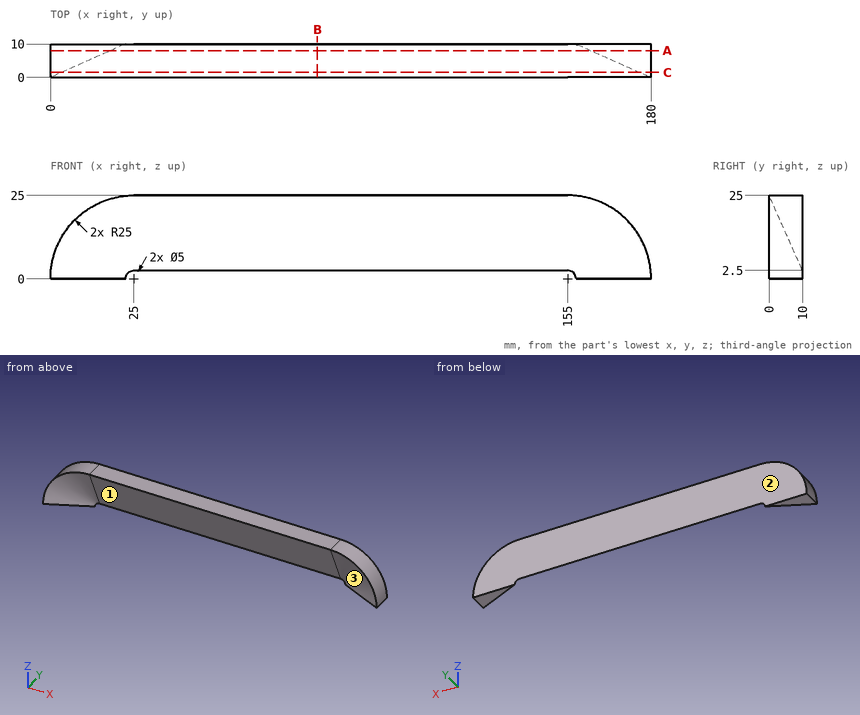
The drawing under review shows one solid part. Ordinate dimensions are in mm from its lowest x, y, z. Give positions to 0.01 mm unless a question says otherwise; leave off trailing zeros. Order: outer loops, then holes, each group sorted by start corner. A loop starts at its lowest first (then second) coordinate and runs counter-clockwise, first axis right, second up. Notation, with made-up numbers: (-33.5, 10) - (0.5, 10) arc R22 cw to (0.5, 27) - close; hole circle Ø1 at (75.25, 25.5). An arc over 180 degrees is marked (long way). Answer as a JSON object with one key per item and string values. Group by question number.
Item 1: Wall thickness on line 1 along X through (y, z) = (1.5, 2.5); line 2 along Y through (x, z) = (92, 15); line 3 along X through (y, z) = (8.75, 21): over which ranges is each line inside the solid? List them lowest first.
Item 2: Draft analysis for pull direction X (two halves, no side actions). For the marked faces 1, 2 and 3, state which applies: pulls with the +X half, pulls with the -X half, needs draft (parallel to the pull), parting line crosses it, or undercut.
Item 3: Take a section at C-C on y = 1.5. Give the boundary of the cut face in (x, z) (3 decimals).
Item 4: Clearance check with flat-ended pins moving along their axes: pin 1 Ø1 at (y, z) = (5.5, 10.5) entering from +X; pin 2 Ø1.5 at (y, z) = (9, 9.5) entering from -X; pin 3 Ø5 at (x, z) = (61.5, 10) entering from -Y. State where each tip first meets the part, or that it passes through.
Item 5: Take a section at A-A on y = 8. Give the boundary of the cut face in (x, z), and give its area (3 significant figures).
Item 6: Take a section at B-B on x = 80. Give the boundary of the cut face in (y, z).
Reported:
{
 "1": {"line 1": "0.13 to 3.52, 176.48 to 179.87", "line 2": "4.44 to 10", "line 3": "11.44 to 168.56"},
 "2": {"face 1": "undercut", "face 2": "needs draft", "face 3": "undercut"},
 "3": {"outline": "(0, 0) - (3.375, 0) arc R21.625 cw to (25, 21.625) - (155, 21.625) arc R21.625 cw to (176.625, 0) - (180, 0) arc R25 ccw to (155, 25) - (25, 25) arc R25 ccw to start"},
 "4": {"pin 1": "x = 177.91", "pin 2": "x = 1.58", "pin 3": "y = 5.56"},
 "5": {"outline": "(0, 0) - (18, 0) arc R7 cw to (25, 7) - (155, 7) arc R7 cw to (162, 0) - (180, 0) arc R25 ccw to (155, 25) - (25, 25) arc R25 ccw to start", "area": "3,240 mm^2"},
 "6": {"outline": "(0, 25) - (10, 2.5) - (10, 25) - close"}
}
